from build123d import *

# Parameters (mm, degrees)
ESQUISSE1_W             = 100
ESQUISSE1_H             = 150
BOSS_EXTRU_1_DEPTH      = 3
ESQUISSE3_R             = 2.4
ENL_V_MAT_EXTRU_2_DEPTH = 3
ESQUISSE4_R             = 1.8
ESQUISSE4_R_2           = 1
ESQUISSE4_W             = 20
ESQUISSE4_H             = 5
ESQUISSE4_W_2           = 26.2
ESQUISSE4_H_2           = 26.2
ESQUISSE4_W_3           = 16.4
ESQUISSE4_H_3           = 35
ESQUISSE4_H_4           = 5.5
ENL_V_MAT_EXTRU_3_DEPTH = 10
CONG_1_R                = 5
CONG_2_R                = 3


with BuildPart() as part:
    # Esquisse1 → Boss.-Extru.1 (new body)
    with BuildSketch(Plane.XY):
        with Locations((50, 75)):
            Rectangle(ESQUISSE1_W, ESQUISSE1_H)
    extrude(amount=BOSS_EXTRU_1_DEPTH)

    # Esquisse3 → Enlèv. mat.-Extru.2 (cut)
    with BuildSketch(Plane.XY.offset(3)):
        with Locations((20, 145)):
            Circle(ESQUISSE3_R)
        with Locations((50, 145)):
            Circle(ESQUISSE3_R)
        with Locations((80, 145)):
            Circle(ESQUISSE3_R)
        with Locations((95, 120)):
            Circle(ESQUISSE3_R)
        with Locations((95, 75)):
            Circle(ESQUISSE3_R)
        with Locations((95, 30)):
            Circle(ESQUISSE3_R)
        with Locations((80, 5)):
            Circle(ESQUISSE3_R)
        with Locations((50, 5)):
            Circle(ESQUISSE3_R)
        with Locations((20, 5)):
            Circle(ESQUISSE3_R)
    extrude(amount=-ENL_V_MAT_EXTRU_2_DEPTH, mode=Mode.SUBTRACT)

    # Esquisse4 → Enlèv. mat.-Extru.3 (cut)
    with BuildSketch(Plane.XY.offset(3)):
        with Locations((44.6, 89.4)):
            Circle(ESQUISSE4_R)
        with Locations((8.4, 125.6)):
            Circle(ESQUISSE4_R)
        with Locations((44.6, 125.6)):
            Circle(ESQUISSE4_R)
        with Locations((85, 128)):
            Circle(ESQUISSE4_R_2)
        with Locations((65, 128)):
            Circle(ESQUISSE4_R_2)
        with Locations((75, 98)):
            Circle(ESQUISSE4_R_2)
        with Locations((8.4, 89.4)):
            Circle(ESQUISSE4_R)
        with Locations((15, 50)):
            Circle(ESQUISSE4_R)
        with Locations((45, 35)):
            Circle(ESQUISSE4_R)
        with Locations((15, 20)):
            Circle(ESQUISSE4_R)
        with Locations((45, 50)):
            Circle(ESQUISSE4_R)
        with Locations((15, 35)):
            Circle(ESQUISSE4_R)
        with Locations((45, 20)):
            Circle(ESQUISSE4_R)
        with Locations((75, 20)):
            Circle(ESQUISSE4_R)
        with Locations((75, 35)):
            Circle(ESQUISSE4_R)
        with Locations((75, 50)):
            Circle(ESQUISSE4_R)
        with BuildLine():
            Line((80, 71), (20, 71))
            ThreePointArc((20, 71), (15, 76), (20, 81))
            Line((20, 81), (80, 81))
            ThreePointArc((80, 81), (85, 76), (80, 71))
        make_face()
        with Locations((30, 42.5)):
            Rectangle(ESQUISSE4_W, ESQUISSE4_H)
        with Locations((60, 42.5)):
            Rectangle(ESQUISSE4_W, ESQUISSE4_H)
        with Locations((60, 27.5)):
            Rectangle(ESQUISSE4_W, ESQUISSE4_H)
        with Locations((30, 27.5)):
            Rectangle(ESQUISSE4_W, ESQUISSE4_H)
        with Locations((26.5, 107.5)):
            Rectangle(ESQUISSE4_W_2, ESQUISSE4_H_2)
        with Locations((59.8, 103.5)):
            Rectangle(ESQUISSE4_W_3, ESQUISSE4_H_3)
        with Locations((30, 14.75)):
            Rectangle(ESQUISSE4_W, ESQUISSE4_H_4)
        with Locations((60, 14.75)):
            Rectangle(ESQUISSE4_W, ESQUISSE4_H_4)
        with BuildLine():
            Line((20, 66), (80, 66))
            ThreePointArc((80, 66), (85, 61), (80, 56))
            Line((80, 56), (20, 56))
            ThreePointArc((20, 56), (15, 61), (20, 66))
        make_face()
        with BuildLine():
            Line((20, 138), (80, 138))
            ThreePointArc((80, 138), (82.5, 135.5), (80, 133))
            Line((80, 133), (20, 133))
            ThreePointArc((20, 133), (17.5, 135.5), (20, 138))
        make_face()
    extrude(amount=-ENL_V_MAT_EXTRU_3_DEPTH, mode=Mode.SUBTRACT)

    # Congé1
    # the kernel refuses this fillet: 5 mm, written as the material it adds along each edge
    with BuildSketch(Plane(origin=(50, 25, 3), x_dir=(0, 1, 0), z_dir=(0, 0, -1)), Plane(origin=(20, 25, 3), x_dir=(0, 1, 0), z_dir=(0, 0, -1)), Plane(origin=(13.4, 94.4, 3), x_dir=(0, 1, 0), z_dir=(0, 0, -1)), Plane(origin=(50, 40, 3), x_dir=(0, 1, 0), z_dir=(0, 0, -1)), Plane(origin=(20, 40, 3), x_dir=(0, 1, 0), z_dir=(0, 0, -1)), Plane(origin=(20, 12, 3), x_dir=(0, 1, 0), z_dir=(0, 0, -1)), Plane(origin=(50, 12, 3), x_dir=(0, 1, 0), z_dir=(0, 0, -1)), Plane(origin=(68, 121, 3), x_dir=(0, -1, 0), z_dir=(0, 0, -1))) as cong_1_piece_1:
        with BuildLine():
            CenterArc((CONG_1_R, CONG_1_R), CONG_1_R, 180, 90)
            Line((0, CONG_1_R), (0, 0))
            Line((0, 0), (CONG_1_R, 0))
        make_face()
    extrude(amount=3)
    with BuildSketch(Plane(origin=(50, 45, 3), x_dir=(0, -1, 0), z_dir=(0, 0, -1)), Plane(origin=(40, 45, 3), x_dir=(-1, 0, 0), z_dir=(0, 0, -1)), Plane(origin=(40, 25, 3), x_dir=(0, 1, 0), z_dir=(0, 0, -1)), Plane(origin=(20, 45, 3), x_dir=(0, -1, 0), z_dir=(0, 0, -1)), Plane(origin=(39.6, 94.4, 3), x_dir=(0, 1, 0), z_dir=(0, 0, -1)), Plane(origin=(39.6, 120.6, 3), x_dir=(-1, 0, 0), z_dir=(0, 0, -1)), Plane(origin=(13.4, 120.6, 3), x_dir=(0, -1, 0), z_dir=(0, 0, -1)), Plane(origin=(70, 40, 3), x_dir=(0, 1, 0), z_dir=(0, 0, -1)), Plane(origin=(70, 45, 3), x_dir=(-1, 0, 0), z_dir=(0, 0, -1)), Plane(origin=(50, 30, 3), x_dir=(0, -1, 0), z_dir=(0, 0, -1)), Plane(origin=(70, 30, 3), x_dir=(-1, 0, 0), z_dir=(0, 0, -1)), Plane(origin=(70, 25, 3), x_dir=(0, 1, 0), z_dir=(0, 0, -1)), Plane(origin=(40, 40, 3), x_dir=(0, 1, 0), z_dir=(0, 0, -1)), Plane(origin=(40, 30, 3), x_dir=(-1, 0, 0), z_dir=(0, 0, -1)), Plane(origin=(20, 30, 3), x_dir=(0, -1, 0), z_dir=(0, 0, -1)), Plane(origin=(20, 17.5, 3), x_dir=(0, -1, 0), z_dir=(0, 0, -1)), Plane(origin=(40, 12, 3), x_dir=(0, 1, 0), z_dir=(0, 0, -1)), Plane(origin=(40, 17.5, 3), x_dir=(-1, 0, 0), z_dir=(0, 0, -1)), Plane(origin=(50, 17.5, 3), x_dir=(0, -1, 0), z_dir=(0, 0, -1)), Plane(origin=(70, 12, 3), x_dir=(0, 1, 0), z_dir=(0, 0, -1)), Plane(origin=(70, 17.5, 3), x_dir=(-1, 0, 0), z_dir=(0, 0, -1)), Plane(origin=(51.6, 86, 3), x_dir=(1, 0, 0), z_dir=(0, 0, -1)), Plane(origin=(68, 86, 3), x_dir=(0, 1, 0), z_dir=(0, 0, -1)), Plane(origin=(51.6, 121, 3), x_dir=(0, -1, 0), z_dir=(0, 0, -1))) as cong_1_piece_2:
        with BuildLine():
            CenterArc((CONG_1_R, -CONG_1_R), CONG_1_R, 90, 90)
            Line((0, -CONG_1_R), (0, 0))
            Line((0, 0), (CONG_1_R, 0))
        make_face()
    extrude(amount=3)

    # Congé2
    cong_2_edges = [part.edges().sort_by_distance(p)[0] for p in [
        (0, 0, 1.5),
        (0, 150, 1.5),
        (100, 150, 1.5),
        (100, 0, 1.5),
    ]]
    fillet(cong_2_edges, radius=CONG_2_R)


solid = part.part
Here's how the part is built. I have some questions about the finished solid (model axes, mm). A direction names the side the tool comes from. Round coordinates to 2 decimals unless told otherwise and drop trailing zeros. Order: outer loops, then holes, each group sorted by start corner. A loop starts at its lowest first (then second) coordinate and runs counter-clockwise, first axis right, second up. Notation, with made-up numbers: M 52,59 L 83,59 A12 cw 83,78 Z; hole C 6.25,-31.5 d3. An arc over 180 degrees is marked long. One line per question, with ' | ' between items.
1) On a 3-axis mill with a long thin cutter (end or side, diameter ignored), from which of +Z, -Z, +X, -X, +Y, -Y can I reach the whole of each face in a straight line? I mean faces 4 (the cylindrical face through (67.589, 16.777, 1.521)), 5 (the flat face through (51, 93, 0)). Say none if no direction works.
Checked values:
face 4: +Z, -Z | face 5: -Z, +X, -X, +Y, -Y
2) Imagine slicing it at C-C, the plane y = 89.4. Write out the boundary of the cut face in (x, z).
Checked values:
outline: M 0,0 L 6.6,0 L 6.6,3 L 0,3 Z; M 10.2,0 L 42.8,0 L 42.8,3 L 10.2,3 Z; M 46.4,0 L 51.86,0 L 51.86,3 L 46.4,3 Z; M 67.74,0 L 100,0 L 100,3 L 67.74,3 Z
3) I'm going to push a flat-ended pin straight in: pin 1 Ø2 at (x, y) = (45, 20) entering from +Z. Where does the tip first touch, or does it pass through?
Checked values:
pin 1: passes through
4) We'd pull the mould along Y, two halves only. Please class faces 1 (the flat face through (60, 17.5, 2)), 2 (the flat face through (51, 93, 3)), 3 (the flat face through (50, 56, 2)): released by +Y, released by -Y, zero draft, split by the parting line, or undercut.
Checked values:
face 1: undercut | face 2: zero draft | face 3: undercut
5) I need wall thicknesses on line 1 (Y direction, x = 50, z = 1.8); line 2 (Y direction, x = 69.5, z = 0.2); line 3 (X direction, y = 116, z = 1.55). Which ranges of each line are inside material? Lowest first, please.
Checked values:
line 1: y = 0 to 2.6, 7.4 to 56, 66 to 71, 81 to 133, 138 to 142.6, 147.4 to 150 | line 2: y = 0 to 56, 66 to 71, 81 to 133, 138 to 150 | line 3: x = 0 to 13.42, 39.58 to 51.6, 68 to 100
6) Imagine slicing it at A-A, the plane x = 26.5. Count the separate pieces of the cut face and the enclosed holes in it, plus the area to 3 significant figures.
Checked values:
separate pieces: 8 | enclosed holes: 0 | area: 250 mm²
7) Imagine slicing it at B-B, the plane y = 113. Write out the boundary of the cut face in (x, z).
Checked values:
outline: M 0,0 L 13.4,0 L 13.4,3 L 0,3 Z; M 39.6,0 L 51.6,0 L 51.6,3 L 39.6,3 Z; M 68,0 L 100,0 L 100,3 L 68,3 Z
8) Imagine slicing it at D-D, the plane y = 135.5. Write out the boundary of the cut face in (x, z), plus the area to 3 significant figures.
Checked values:
outline: M 0,0 L 17.5,0 L 17.5,3 L 0,3 Z; M 82.5,0 L 100,0 L 100,3 L 82.5,3 Z | area: 105 mm²
